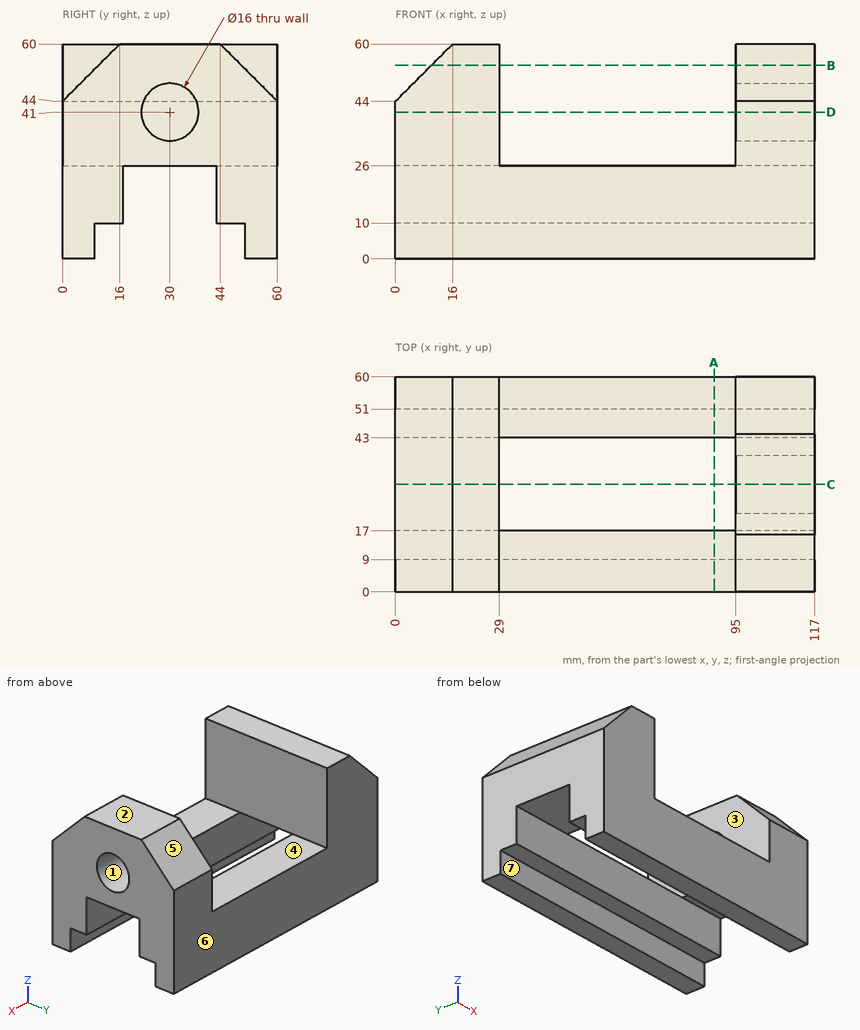
Could you check a few things on this drawing? It's one solid part, dimensions in mm from its lowest x, y, z. A direction names the side the tool comes from. Round coordinates to 2 decimals unless told otherwise and drop trailing zeros. Write each loop counter-clockwise with the first axis right and the second up, starting at its lowest first coordinate (ties: lowest second). Pieces come first, ordered by that corner, then holes.
Q1. Which directions (+Z, -Z, +X, -X, +Y, -Y) give clear straight access to the entire face, cutting with the end or side of a thin tool? Please do the marked faces 4, 5, 6 and 7.
Q2. If we section it at D-D on z = 41: Write out the boundary of the cut face in (x, y).
Q3. If we mould it in two halves opening along Z, with no side actions, what happens to the marked faces 1, 2 and 3? For each: +Z half, -Z half, draft (parallel to the pull), parting line (faces both ways), or undercut.
Q4. If we section it at B-B on z = 54: Write out the boundary of the cut face in (x, y), plus the area to 3 significant figures.
Q5. Please list where these lines run through material, in increasing order: probe 1 along Z at (x, y) = (111.75, 30); probe 2 along X at (y, z) = (11.5, 36.5); probe 3 along Y at (x, z) = (62.5, 22.5).
Q6. If we section it at C-C on y = 30: Write out the boundary of the cut face in (x, z).
Q7. If we section it at A-A on x = 89: Write out the boundary of the cut face in (y, z).
Q8. Will these pins go through, and if not, where does the flat tip stop? P1, Ø11, axis at x = 104, y = 33, coming from the -Z side; P2, Ø21, axis at x = 16, y = 36, coming from the -Z side; P3, Ø5, axis at x = 58.5, y = 6.5, coming from the +Z side.
Answer below:
1. face 4: +Z, +Y, -Y
1. face 5: +Z, +X, +Y
1. face 6: +Z, -Z, +X, -X, +Y
1. face 7: -Z, +X, -X
2. outline: (0, 0) - (29, 0) - (29, 60) - (0, 60) - close; (95, 0) - (117, 0) - (117, 22) - (95, 22) - close; (95, 38) - (117, 38) - (117, 60) - (95, 60) - close
3. face 1: undercut
3. face 2: +Z half
3. face 3: draft
4. outline: (10, 0) - (29, 0) - (29, 60) - (10, 60) - close; (95, 10) - (117, 10) - (117, 50) - (95, 50) - close
4. area: 2,020 mm2
5. probe 1: z = 26 to 33, 49 to 60
5. probe 2: x = 0 to 29, 95 to 117
5. probe 3: y = 0 to 17, 43 to 60
6. outline: (0, 26) - (29, 26) - (29, 60) - (16, 60) - (0, 44) - close; (95, 26) - (117, 26) - (117, 33) - (95, 33) - close; (95, 49) - (117, 49) - (117, 60) - (95, 60) - close
7. outline: (0, 0) - (9, 0) - (9, 10) - (17, 10) - (17, 26) - (0, 26) - close; (43, 10) - (51, 10) - (51, 0) - (60, 0) - (60, 26) - (43, 26) - close
8. P1: stops at z = 26
8. P2: stops at z = 10
8. P3: stops at z = 26
